```python
from build123d import *

# Parameters (mm, degrees)
SKETCH1_W           = 65
SKETCH1_H           = 70
BOSS_EXTRUDE1_DEPTH = 25
SKETCH8_W           = 61
SKETCH8_H           = 21
CUT_EXTRUDE1_DEPTH  = 40
SKETCH9_R           = 2.5
CUT_EXTRUDE2_DEPTH  = 30


with BuildPart() as part:
    # Sketch1 → Boss-Extrude1 (new body)
    with BuildSketch(Plane(origin=(0, 0, 0), x_dir=(1, 0, 0), z_dir=(0, 1, 0))):
        with Locations((32.5, -35)):
            Rectangle(SKETCH1_W, SKETCH1_H)
    extrude(amount=BOSS_EXTRUDE1_DEPTH)

    # Sketch8 → Cut-Extrude1 (cut)
    with BuildSketch(Plane(origin=(0, 0, 0), x_dir=(-1, 0, 0), z_dir=(0, 0, -1))):
        with Locations((-32.5, 12.5)):
            Rectangle(SKETCH8_W, SKETCH8_H)
    extrude(amount=-CUT_EXTRUDE1_DEPTH, mode=Mode.SUBTRACT)

    # Sketch9 → Cut-Extrude2 (cut)
    with BuildSketch(Plane(origin=(0, 25, 0), x_dir=(1, 0, 0), z_dir=(0, 1, 0))):
        with Locations(Location((32.5, -20, 0), (0, 0, 270))):
            Circle(SKETCH9_R)
    extrude(amount=-CUT_EXTRUDE2_DEPTH, mode=Mode.SUBTRACT)


solid = part.part
```
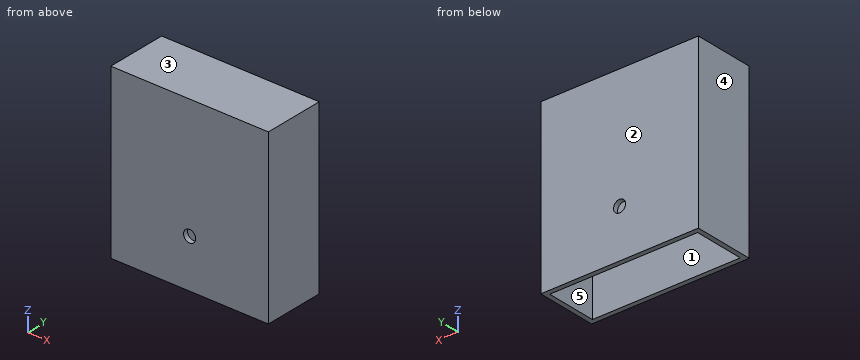
The listing builds one solid part. Answer for the finished solid, in the listing's coordinates (mm). Face numbers are marked on the shaded views. A direction names the side the tool comes from. Give positions to 0.01 mm unless a question says otherwise; leave off trailing zeros. Order: outer loops, then holes, each group sorted by start corner. A loop starts at its lowest first (then second) coordinate and runs counter-clockwise, first axis right, second up. Notation, with made-up numbers: (56.5, 68) -> (96.5, 68) arc R23 ccw to (96.5, 78) -> close; hole circle Ø9 at (13.25, -36.5). An arc over 180 degrees is marked (long way). One line per item, written item: value.
1) Find section C-C, the plane z = 37. Determine the outline of the cut face in (x, y).
Reported:
outline: (0, 0) -> (65, 0) -> (65, 25) -> (0, 25) -> close; hole (2, 2) -> (63, 2) -> (63, 23) -> (2, 23) -> close
2) Find section A-A, the plane z = 20. Determine the outline of the cut face in (x, y), plus the area to 3 significant figures.
Reported:
outline: (0, 0) -> (30, 0) -> (30, 2) -> (2, 2) -> (2, 23) -> (30, 23) -> (30, 25) -> (0, 25) -> close; (35, 0) -> (65, 0) -> (65, 25) -> (35, 25) -> (35, 23) -> (63, 23) -> (63, 2) -> (35, 2) -> close
area: 324 mm^2
3) A flat-ended cylindrical pin translates along its axis: P1, Ø6, axis at x = 32.5, z = 20, coming from the -Y side. Find the tip coordinate at first contact, or state that the pin passes through.
Reported:
P1: stops at y = 0
4) Find section B-B, the plane x = 32.5. Determine the outline of the cut face in (y, z), plus the area to 3 significant figures.
Reported:
outline: (0, 0) -> (2, 0) -> (2, 17.5) -> (0, 17.5) -> close; (0, 22.5) -> (2, 22.5) -> (2, 40) -> (23, 40) -> (23, 22.5) -> (25, 22.5) -> (25, 70) -> (0, 70) -> close; (23, 0) -> (25, 0) -> (25, 17.5) -> (23, 17.5) -> close
area: 890 mm^2
5) Find section D-D, the plane x = 16.5. Determine the outline of the cut face in (y, z).
Reported:
outline: (0, 0) -> (2, 0) -> (2, 40) -> (23, 40) -> (23, 0) -> (25, 0) -> (25, 70) -> (0, 70) -> close
6) Determine the mould class of the marked faces 3, 4 and 5 for opening direction X: pulls with the +X half, pulls with the -X half, needs draft (parallel to the pull), parting line crosses it, or undercut.
Reported:
face 3: needs draft
face 4: pulls with the -X half
face 5: undercut
7) Find the intervals of material crossed by line 1 (X direction, y = 21, z = 38.5); line 2 (Y direction, x = 57, z = 9.5); line 3 (X direction, y = 24.45, z = 20), in increasing order.
Reported:
line 1: x = 0 to 2, 63 to 65
line 2: y = 0 to 2, 23 to 25
line 3: x = 0 to 30, 35 to 65
8) A tool of negligible diameter and unlimited length cuts with its end or side. For the marked faces 1 and 2, from which of +Z, -Z, +X, -X, +Y, -Y can it reach the whole face along a straight path? Write none if from no direction.
Reported:
face 1: -Z
face 2: +Z, -Z, +X, -X, +Y
